Job drawing, mm, ordinate dimensions from the low corner. One solid piece. A direction names the side the tool comes from. Give positions to 0.01 mm unless a question says otherwise; leave off trailing zeros. Order: outer loops, then holes, each group sorted by start corner. A loop starts at its lowest first (then second) coordinate and runs counter-clockwise, first axis right, second up. Notation, with made-up numbers: M 55,65 L 83,65 A16 cw 83,89 Z; hole C 62,89.5 d1. An arc over 180 degrees is marked long. One line per question, with ' | ' between items.
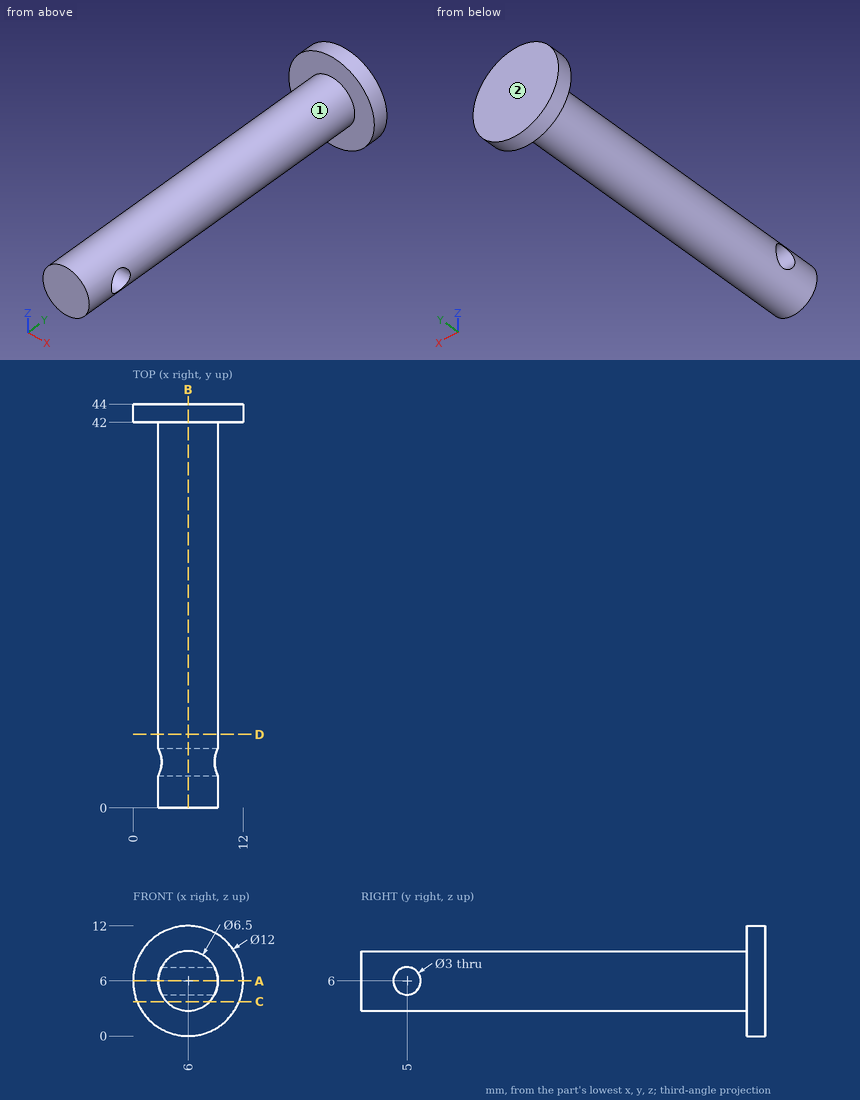
1. Slice it at C-C on z = 3.75. Give the cut face in (x, y).
Worked out:
outline: M 0.44,42 L 3.65,42 L 3.65,0 L 8.35,0 L 8.35,42 L 11.56,42 L 11.56,44 L 0.44,44 Z
2. Slice it at B-B on x = 6. Give the cut face in (y, z), then the cut area to 3 significant figures.
Worked out:
outline: M 0,2.75 L 42,2.75 L 42,0 L 44,0 L 44,12 L 42,12 L 42,9.25 L 0,9.25 Z; hole C 5,6 d3 | area: 290 mm2
3. Drop flat-ended pins along their axis: pin 1 (2 mm diameter, centred on y = 20.5, z = 7, fed in from -X); pin 2 (1.8 mm diameter, centred on y = 5, z = 6, fed in from -X); pin 3 (1 mm diameter, centred on x = 3, y = 5.5, fed in from -Z); pin 4 (1 mm diameter, centred on y = 31.5, z = 3, fed in from -X). Give the stop position or say it passes through.
Worked out:
pin 1: stops at x = 2.75 | pin 2: passes through | pin 3: stops at z = 3.92 | pin 4: stops at x = 3.92
4. Tool access for the marked faces 1 and 2: list every direction of +Z, -Z, +X, -X, +Y, -Y with a clear straight run to the whole face (end or side of a thin tool).
Worked out:
face 1: -Y | face 2: +Z, -Z, +X, -X, +Y
5. Slice it at D-D on y = 8. Give the cut face in (x, z).
Worked out:
outline: C 6,6 d6.5
6. Probe L1, parallel to Y at x = 4.5, z = 6; L2, parallel to Y at x = 7.25, z = 9.25; L3, parallel to Z at x = 5.5, y = 5. List the from-to ranges inside material, lowest first. Write a range as from..to.
Worked out:
L1: y = 0..3.5, 6.5..44 | L2: y = 42..44 | L3: z = 2.79..4.5, 7.5..9.21
7. Slice it at A-A on z = 6. Give the cut face in (x, y).
Worked out:
outline: M 0,42 L 2.75,42 L 2.75,6.5 L 9.25,6.5 L 9.25,42 L 12,42 L 12,44 L 0,44 Z; M 2.75,0 L 9.25,0 L 9.25,3.5 L 2.75,3.5 Z
